from build123d import *

# Parameters (mm, degrees)
SKETCH1_W               = 8
SKETCH1_H               = 8
BOSS_EXTRUDE1_DEPTH     = 3
CUT_EXTRUDE1_DEPTH      = 12.704699911
CUT_EXTRUDE1_DEPTH_BACK = 12.704699911
CUT_EXTRUDE2_DEPTH      = 11
SKETCH4_R               = 1.8
CUT_EXTRUDE3_DEPTH      = 0.8
SKETCH5_W               = 8
SKETCH5_H               = 1
BOSS_EXTRUDE2_DEPTH     = 2
FILLET1_R               = 4
CUT_EXTRUDE4_DEPTH      = 0.4
CUT_EXTRUDE5_DEPTH      = 0.4


with BuildPart() as part:
    # Sketch1 → Boss-Extrude1 (new body)
    with BuildSketch(Plane(origin=(0, 0, 0), x_dir=(1, 0, 0), z_dir=(0, 1, 0))):
        with Locations((4, 4)):
            Rectangle(SKETCH1_W, SKETCH1_H)
    extrude(amount=BOSS_EXTRUDE1_DEPTH)

    # Sketch2 → Cut-Extrude1 (cut, two sides: drawn at the far end of the back side and taken through both)
    with BuildSketch(Plane.XY.offset(-CUT_EXTRUDE1_DEPTH_BACK)):
        Polygon((0, 0), (0.6, 3), (0, 3), align=None)
        Polygon((8, 0), (7.4, 3), (8, 3), align=None)
    extrude(amount=CUT_EXTRUDE1_DEPTH + CUT_EXTRUDE1_DEPTH_BACK, mode=Mode.SUBTRACT)

    # Sketch3 → Cut-Extrude2 (cut)
    with BuildSketch(Plane(origin=(0, 0, 0), x_dir=(0, 0, -1), z_dir=(1, 0, 0))):
        Polygon((0, 0), (0.6, 3), (0, 3), align=None)
        Polygon((8, 3), (7.4, 3), (8, 0), align=None)
    extrude(amount=CUT_EXTRUDE2_DEPTH, mode=Mode.SUBTRACT)

    # Sketch4 → Cut-Extrude3 (cut)
    with BuildSketch(Plane.XZ):
        with Locations(Location((4, -3.75, 0), (0, 0, 270))):
            Circle(SKETCH4_R)
    extrude(amount=-CUT_EXTRUDE3_DEPTH, mode=Mode.SUBTRACT)

    # Sketch5 → Boss-Extrude2 (add)
    with BuildSketch(Plane.XZ):
        with Locations((4, -7.5)):
            Rectangle(SKETCH5_W, SKETCH5_H)
    extrude(amount=BOSS_EXTRUDE2_DEPTH)

    # Fillet1
    # the kernel refuses this fillet: 4 mm, written as the material it takes off along each edge
    with BuildSketch(Plane(origin=(8, -2, -16.660254038), x_dir=(0, 1, 0), z_dir=(0, 0, 1)), Plane(origin=(0, -2, 1.660254038), x_dir=(0, 1, 0), z_dir=(0, 0, -1))) as fillet1_piece_1:
        with BuildLine():
            CenterArc((4, 3.464101615), FILLET1_R, 180, 60)
            Line((0, 3.464101615), (-0.08, 3.464101615))
            Line((-0.08, 3.464101615), (-0.08, 0))
            Line((-0.08, 0), (0, -0.08))
            ThreePointArc((0, -0.08), (1, -0.08), (1.96, -0.069282032))
            Line((1.96, -0.069282032), (2, 0))
        make_face()
    extrude(amount=18.320508076, mode=Mode.SUBTRACT)

    # Sketch6 → Cut-Extrude4 (cut)
    with BuildSketch(Plane(origin=(0, 3, 0), x_dir=(1, 0, 0), z_dir=(0, 1, 0))):
        Polygon((3.623842243, 2.056832464), (3.623842243, 3.740326053), (2.162303782, 6.056832464), (3.062143525, 6.056832464), (4.007656346, 4.408595284), (4.95477173, 6.056832464), (5.854611474, 6.056832464), (4.393073013, 3.734717079), (4.393073013, 2.056832464), align=None)
    extrude(amount=-CUT_EXTRUDE4_DEPTH, mode=Mode.SUBTRACT)

    # Sketch7 → Cut-Extrude5 (cut)
    with BuildSketch(Plane(origin=(0, 3, 0), x_dir=(1, 0, 0), z_dir=(0, 1, 0))):
        with BuildLine():
            Line((6.99657775, 2.307478491), (6.650423904, 2.269617914))
            add(Edge.make_bspline(
                [(6.650423904, 2.269617914), (6.648104786, 2.286290214), (6.643740629, 2.317664439), (6.630814222, 2.360960848), (6.6128192, 2.397384178), (6.589720846, 2.426985356), (6.562208273, 2.449767653), (6.53085918, 2.465955864), (6.495693494, 2.475565581), (6.471038508, 2.476713937), (6.458236404, 2.477310221)],
                knots=[0, 0, 0, 0, 1.280716388, 2.410074291, 3.425374506, 4.35753932, 5.248331359, 6.12451615, 7.026154803, 8, 8, 8, 8], degree=3))
            add(Edge.make_bspline(
                [(6.458236404, 2.477310221), (6.449554942, 2.477097941), (6.432279271, 2.476675513), (6.407115159, 2.471312362), (6.382853927, 2.463353411), (6.359693582, 2.452081234), (6.337518567, 2.437536581), (6.316665994, 2.419545601), (6.296177185, 2.39905664), (6.277258092, 2.37431526), (6.259107425, 2.34501973), (6.243478966, 2.309156475), (6.229549311, 2.266758815), (6.217622545, 2.217619097), (6.206799126, 2.162049229), (6.197926997, 2.099824257), (6.190827571, 2.030888275), (6.1874217, 1.982610246), (6.18564025, 1.957358298)],
                knots=[0, 0, 0, 0, 0.642458078, 1.278459126, 1.898279436, 2.531842133, 3.181731979, 3.858193002, 4.57010051, 5.325711302, 6.161524323, 7.118599443, 8.217371811, 9.466325973, 10.864147948, 12.412648259, 14.123626419, 16, 16, 16, 16], degree=3))
            add(Edge.make_bspline(
                [(6.18564025, 1.957358298), (6.196703374, 1.969374309), (6.218396997, 1.992936442), (6.254393564, 2.023656049), (6.292105324, 2.049919261), (6.331942634, 2.071465901), (6.374122941, 2.087500286), (6.417882183, 2.099674887), (6.463793169, 2.1064945), (6.494994081, 2.107544715), (6.510880634, 2.108079452)],
                knots=[0, 0, 0, 0, 1.057745406, 2.074127497, 3.059409796, 4.031705469, 5.000875988, 5.977809597, 6.970362319, 8, 8, 8, 8], degree=3))
            add(Edge.make_bspline(
                [(6.510880634, 2.108079452), (6.528809934, 2.107563089), (6.564213931, 2.106543456), (6.616372239, 2.099391957), (6.666421561, 2.086532277), (6.714588312, 2.069136373), (6.761110551, 2.047230594), (6.805098359, 2.019501147), (6.847242227, 1.987169858), (6.886962554, 1.950231753), (6.923455982, 1.909566001), (6.95567607, 1.865643773), (6.982192143, 1.818330938), (7.00486021, 1.76868676), (7.021726117, 1.715731209), (7.033968982, 1.660226315), (7.04127711, 1.601662587), (7.042239139, 1.561706039), (7.042731596, 1.541252529)],
                knots=[0, 0, 0, 0, 0.99135015, 1.957564468, 2.903754199, 3.843479786, 4.78583385, 5.741106244, 6.712813504, 7.719198368, 8.735844933, 9.730198001, 10.724351158, 11.729813921, 12.742848014, 13.790983496, 14.86921809, 16, 16, 16, 16], degree=3))
            add(Edge.make_bspline(
                [(7.042731596, 1.541252529), (7.042231952, 1.519599685), (7.041257525, 1.477371451), (7.034085066, 1.415527203), (7.021415455, 1.357153196), (7.004106031, 1.301781092), (6.981716795, 1.249849655), (6.954594052, 1.200930916), (6.921819947, 1.155860856), (6.884881845, 1.114033218), (6.84370317, 1.076707467), (6.799818397, 1.043655074), (6.752740779, 1.016179585), (6.703166183, 0.993054256), (6.650243128, 0.9760833), (6.594904638, 0.963355935), (6.536700741, 0.955593381), (6.496962304, 0.954693712), (6.476625827, 0.954233298)],
                knots=[0, 0, 0, 0, 1.13287417, 2.209376133, 3.25169942, 4.254157582, 5.240146322, 6.205890558, 7.174579019, 8.150183866, 9.1206468, 10.07783463, 11.019441811, 11.967766696, 12.934309213, 13.921380422, 14.936249089, 16, 16, 16, 16], degree=3))
            add(Edge.make_bspline(
                [(6.476625827, 0.954233298), (6.454835686, 0.954842926), (6.411992392, 0.956041562), (6.349274568, 0.965905733), (6.289647802, 0.982594351), (6.233119501, 1.005900716), (6.179219819, 1.035216515), (6.128449255, 1.071632083), (6.080942348, 1.114800151), (6.036070744, 1.164136126), (5.995238787, 1.221123075), (5.960465944, 1.286988003), (5.930975089, 1.361009558), (5.906965213, 1.443377578), (5.888431321, 1.534085529), (5.875498792, 1.633141016), (5.86690889, 1.740380226), (5.866183985, 1.814672002), (5.865808519, 1.853151567)],
                knots=[0, 0, 0, 0, 0.852151446, 1.675481364, 2.476404467, 3.269281233, 4.062617998, 4.871616733, 5.707301388, 6.56955125, 7.476395267, 8.442009786, 9.475854496, 10.58877921, 11.794095973, 13.094195288, 14.494932947, 16, 16, 16, 16], degree=3))
            add(Edge.make_bspline(
                [(5.865808519, 1.853151567), (5.866346697, 1.892590697), (5.867386586, 1.968796599), (5.875754473, 2.078827487), (5.889046125, 2.180436336), (5.908408745, 2.273394012), (5.933175033, 2.357893394), (5.963200156, 2.434104295), (5.99923844, 2.501750812), (6.041138584, 2.560612949), (6.087240817, 2.61177964), (6.136777869, 2.655945181), (6.189560624, 2.693536639), (6.245587817, 2.724459089), (6.305319384, 2.747901225), (6.368188753, 2.764829378), (6.434301522, 2.775708833), (6.479587723, 2.776770851), (6.502587365, 2.777310221)],
                knots=[0, 0, 0, 0, 1.491699013, 2.882321987, 4.171520357, 5.365488089, 6.470299549, 7.49861535, 8.458736801, 9.361983288, 10.224742848, 11.058789056, 11.867429157, 12.671146298, 13.473202851, 14.288259215, 15.130652936, 16, 16, 16, 16], degree=3))
            add(Edge.make_bspline(
                [(6.502587365, 2.777310221), (6.518832845, 2.777017956), (6.550590682, 2.776446616), (6.597136362, 2.770379458), (6.641540508, 2.76110179), (6.683919501, 2.748259344), (6.723974963, 2.731060825), (6.761865954, 2.710109046), (6.797719857, 2.685460752), (6.831350121, 2.657274635), (6.862486078, 2.625465393), (6.890601127, 2.589961055), (6.915881459, 2.551190115), (6.938437714, 2.509184749), (6.957357529, 2.46354265), (6.973622233, 2.414622738), (6.98699882, 2.362319913), (6.993336088, 2.326037695), (6.99657775, 2.307478491)],
                knots=[0, 0, 0, 0, 1.036027791, 2.025301876, 2.989435482, 3.928225244, 4.845595412, 5.765526461, 6.686607585, 7.61747015, 8.561102691, 9.521661062, 10.50224679, 11.510949117, 12.559251378, 13.650572309, 14.798212656, 16, 16, 16, 16], degree=3))
        make_face()
        with BuildLine():
            add(Edge.make_bspline(
                [(6.211962365, 1.549185221), (6.212093793, 1.537753077), (6.212350595, 1.515415322), (6.216561681, 1.483001611), (6.222614755, 1.452614338), (6.230767911, 1.42408476), (6.242068736, 1.397844656), (6.255476173, 1.373367715), (6.271335314, 1.350875727), (6.295669246, 1.324486058), (6.329294099, 1.29676891), (6.373421783, 1.272086886), (6.420703408, 1.256744198), (6.453316703, 1.255075433), (6.469774865, 1.254233298)],
                knots=[0, 0, 0, 0, 0.93816693, 1.833124408, 2.679057427, 3.481731691, 4.264557977, 5.020023694, 5.770442996, 6.518065735, 7.962605608, 9.32780964, 10.651490302, 12, 12, 12, 12], degree=3))
            add(Edge.make_bspline(
                [(6.469774865, 1.254233298), (6.485365796, 1.254933043), (6.51571185, 1.256295021), (6.559046727, 1.268742487), (6.598409917, 1.288373431), (6.627266187, 1.311420354), (6.647387039, 1.333836313), (6.660907792, 1.353494474), (6.671913698, 1.375919542), (6.680911589, 1.400742183), (6.688159323, 1.427866383), (6.693107691, 1.457564676), (6.69591447, 1.48975573), (6.696351403, 1.512040132), (6.69657775, 1.52358426)],
                knots=[0, 0, 0, 0, 1.399678333, 2.724321989, 4.020062797, 5.33532049, 6.016755754, 6.724441967, 7.473839083, 8.257094862, 9.096253071, 9.995581596, 10.961638663, 12, 12, 12, 12], degree=3))
            add(Edge.make_bspline(
                [(6.69657775, 1.52358426), (6.696384678, 1.535490976), (6.696011412, 1.558510238), (6.692745041, 1.591780733), (6.687401372, 1.622537963), (6.679930507, 1.650999261), (6.669817892, 1.676783929), (6.657887501, 1.700412041), (6.643402955, 1.721242874), (6.621876525, 1.745742616), (6.590576263, 1.770429427), (6.548753213, 1.792915191), (6.501874013, 1.805662518), (6.469248141, 1.807258544), (6.452467173, 1.808079452)],
                knots=[0, 0, 0, 0, 1.008384627, 1.949510571, 2.828269698, 3.650667555, 4.437180943, 5.170285793, 5.887596972, 6.580056709, 7.926803404, 9.238379296, 10.579573008, 12, 12, 12, 12], degree=3))
            add(Edge.make_bspline(
                [(6.452467173, 1.808079452), (6.436151813, 1.807414866), (6.404464825, 1.806124136), (6.358926875, 1.793162443), (6.31725918, 1.772538153), (6.286568407, 1.748308757), (6.264936989, 1.725473324), (6.25076935, 1.706030549), (6.238437114, 1.684862342), (6.228698053, 1.661421349), (6.221189386, 1.636147459), (6.215803903, 1.608867965), (6.212544961, 1.579673333), (6.212160051, 1.559530412), (6.211962365, 1.549185221)],
                knots=[0, 0, 0, 0, 1.469034193, 2.853094746, 4.235454457, 5.641396914, 6.354997179, 7.06867986, 7.807229614, 8.560602297, 9.353235934, 10.182779392, 11.06669468, 12, 12, 12, 12], degree=3))
        make_face(mode=Mode.SUBTRACT)
    extrude(amount=-CUT_EXTRUDE5_DEPTH, mode=Mode.SUBTRACT)


solid = part.part
Input: part model. Units: mm. Frame: model coordinates. A direction names the side the tool comes from. Give positions to 0.01 mm unless a question says otherwise; leave off trailing zeros. Order: outer loops, then holes, each group sorted by start corner. A loop starts at its lowest first (then second) coordinate and runs counter-clockwise, first axis right, second up. Notation, with made-up numbers: M 60.25,-31 L 67.25,-31 A33 ccw 67.25,8 Z; hole C 30,2 d4. An arc over 180 degrees is marked long. Answer as a JSON object with one key per item and string values.
1. Ray query, line 1 (Z direction, x = 1.5, y = -0.65); line 2 (Y direction, x = 4, z = -6.25); line 3 (Y direction, x = 4.25, z = -2). Return the intervals inside material, ascending. Write a range as [from, to].
Result sheet:
{"line 1": "[-8, -7]", "line 2": "[0, 3]", "line 3": "[0.8, 3]"}
2. Reachability of faces 1 (the flat face through (4, -1, -7)), 2 (the cylindrical face through (6.51, -1.48, -7.51)), 3 (the flat face through (4, 0.8, -4)), 4 (the cylindrical face through (1.49, -1.48, -7.49)), 5 (the flat face through (5.134, 2.803, -4.912)) from +Z, -Z, +X, -X, +Y, -Y: full face, straight path, thin tool, end or side. Return the list, or none.
Result sheet:
{"face 1": "+Z, +X, -X, -Y", "face 2": "+Z, -Z, +X, -Y", "face 3": "-Y", "face 4": "+Z, -Z, -X, -Y", "face 5": "+Y"}
3. Cut plane C-C, the plane z = -3.5. Output: boundary loops of the cut face in (x, y).
Result sheet:
{"outline": "M 0,0 L 2.22,0 L 2.22,0.8 L 5.78,0.8 L 5.78,0 L 8,0 L 7.4,3 L 4.39,3 L 4.39,2.6 L 3.62,2.6 L 3.62,3 L 0.6,3 Z"}
4. Cut plane A-A, the plane y = 0.5. Output: boundary loops of the cut face in (x, z), and give its area (3 significant figures).
Result sheet:
{"outline": "M 0.1,-7.9 L 7.9,-7.9 L 7.9,-0.1 L 0.1,-0.1 Z; hole C 4,-3.75 d3.6", "area": "50.7 mm²"}
5. Cut plane B-B, the plane x = 0.5. Output: boundary loops of the cut face in (y, z).
Result sheet:
{"outline": "M -0.69,-8 L 0,-8 L 2.5,-7.5 L 2.5,-0.5 L 0,0 L 0,-7 L -0.69,-7 Z"}
6. Cut plane D-D, the plane x = 4.25. Output: boundary loops of the cut face in (y, z).
Result sheet:
{"outline": "M -2,-8 L 0,-8 L 3,-7.4 L 3,-4.83 L 2.6,-4.83 L 2.6,-2.06 L 3,-2.06 L 3,-0.6 L 0,0 L 0,-1.97 L 0.8,-1.97 L 0.8,-5.53 L 0,-5.53 L 0,-7 L -2,-7 Z"}
7. Pull-direction query (X, two-part tool) for faces 6 (the cylindrical face through (4.541, 0.394, -5.467)), 7 (the flat face through (4, -2, -7.5)), 8 (the flat face through (0.3, 1.5, -4.1)), 9 (the flat face through (4.475, 2.803, -5.221)); classes: +X half, -X half, draft (parallel to the pull), parting line (faces both ways), or undercut.
Result sheet:
{"face 6": "undercut", "face 7": "draft", "face 8": "-X half", "face 9": "undercut"}
8. First-contact query: P1, Ø3, axis at y = 1.5, z = -7, coming from the -X side; P2, Ø1, axis at x = 5, y = -1, coming from the +Z side; P3, Ø3, axis at x = 4.5, z = -4.5, coming from the -Y side. Flat tips, straight axial feed; report the tip coordinate or a pass-through.
Result sheet:
{"P1": "x = 0", "P2": "z = -7", "P3": "y = 0"}
